```python
from build123d import *

# Parameters (mm, degrees)
F0_W           = 92.075
F0_H           = 22.225
F0_R           = 6.35
F1_DEPTH       = 6.35
F3_D           = 1.5875
F3_CSINK_D     = 6.35
F3_CSINK_ANGLE = 90
F6_D           = 12.7
F6_CBORE_D     = 19.05
F6_CBORE_DEPTH = 4.7625
F7_SIZE2       = 25.4
F7_SIZE        = 6.35
F8_R           = 3.175
F9_R           = 1.5875


with BuildPart() as f1:
    # F0 (on Top) → F1 (new body)
    with BuildSketch(Plane.XY):
        Rectangle(F0_W, F0_H)
        Circle(F0_R, mode=Mode.SUBTRACT)
    extrude(amount=-F1_DEPTH)

    # F3 (through all)
    with Locations(Plane.XY):
        with Locations((26.9875, 0), (-26.9875, 0)):
            CounterSinkHole(F3_D / 2, F3_CSINK_D / 2, counter_sink_angle=F3_CSINK_ANGLE)

    # F6 (through all)
    with Locations(Plane(origin=(0, 0, -6.35), x_dir=(1, 0, 0), z_dir=(0, 0, -1))):
        with Locations((0, 0)):
            CounterBoreHole(F6_D / 2, F6_CBORE_D / 2, F6_CBORE_DEPTH)

    # F7
    f7_edges = [f1.edges().sort_by_distance(p)[0] for p in [
        (-46.0375, -11.1125, -3.175),
        (-46.0375, 11.1125, -3.175),
    ]]
    f7_side = f1.faces().sort_by_distance((-46.0375, 0, -3.175))[0]
    chamfer(f7_edges, length=F7_SIZE, length2=F7_SIZE2, reference=f7_side)

    # F8
    f8_edges = [f1.edges().sort_by_distance(p)[0] for p in [
        (-46.0375, -4.7625, -3.175),
        (-46.0375, 4.7625, -3.175),
    ]]
    fillet(f8_edges, radius=F8_R)

    # F9
    f9_edges = [f1.edges().sort_by_distance(p)[0] for p in [
        (12.7, -11.1125, 0),
        (46.0375, 0, 0),
        (12.7, 11.1125, 0),
        (-32.135025, -8.238119, 0),
        (-32.135025, 8.238119, 0),
        (-45.365052, 4.237469, 0),
        (-46.0375, 0, 0),
        (-45.365052, -4.237469, 0),
        (46.0375, -11.1125, -3.175),
        (46.0375, 11.1125, -3.175),
    ]]
    fillet(f9_edges, radius=F9_R)


solid = f1.part
```
Geometry check sheet. Reference: the model listing, model coordinates, mm. Round coordinates to 2 decimals unless told otherwise and drop trailing zeros. Use a Markdown table: item, result.
Q1. Cross-section at A-A on y = 0. State how many separate pieces and enclosed holes the cut face has, plus the area to 3 significant figures.
Solutions:
| item | result |
|---|---|
| separate pieces | 4 |
| enclosed holes | 0 |
| area | 441 mm2 |
Q2. Go/stop test with flat-tipped pins: P1, Ø1.5, axis at x = -35, z = -2, coming from the -Y side; P2, Ø2, axis at x = -32, z = -5, coming from the -Y side; P3, Ø5.5, axis at x = 1, y = -0.5, coming from the -Z side; P4, Ø1, axis at x = -27, z = -1, coming from the +Y side. Record where each tip stops, or that it passes through.
Solutions:
| item | result |
|---|---|
| P1 | stops at y = -7.71 |
| P2 | stops at y = -8.52 |
| P3 | passes through |
| P4 | stops at y = 9.59 |
Q3. Draft check along Y on faces 1 (the cylindrical face through (-31.858, -7.815, -0.453)), 2 (the cylindrical face through (-27.745, 0.238, -4.393)), 3 (the flat face through (-46.038, 0, -4)), 4 (the cylindrical face through (-1.38, -6.2, -0.78)). Enter one of: released by +Y, released by -Y, zero draft, split by the parting line, or undercut.
Solutions:
| item | result |
|---|---|
| face 1 | released by -Y |
| face 2 | undercut |
| face 3 | zero draft |
| face 4 | undercut |
Q4. Material ranges on line 1 (X direction, y = 0, z = -0.95); line 2 (Y direction, x = 0, z = -3.15) (1 decimal); line 3 (Y direction, x = -4, z = -1), recorded low to high.
Solutions:
| item | result |
|---|---|
| line 1 | x = -45.9 to -29.21, -24.76 to -6.35, 6.35 to 24.76, 29.21 to 45.9 |
| line 2 | y = -11.1 to -9.5, 9.5 to 11.1 |
| line 3 | y = -11 to -4.93, 4.93 to 11 |
